Here's how the part is built. I have some questions about the finished solid (model axes, mm). A direction names the side the tool comes from. Round coordinates to 2 decimals unless told otherwise and drop trailing zeros. Loops run counter-clockwise (first coordinate to the right, second up) from the corner with the lowest first, then second, coordinate; pieces in that order, holes last. Notation, with made-up numbers: M -6.75,-12.5 L 28.25,-12.5 A34 cw 28.25,24.5 Z; hole C -33.75,59 d3. An arc over 180 degrees is marked long. Write item = value, one per line. Start each with the question number.
from build123d import *

# Parameters (mm, degrees)
F3_W         = 3.5
F3_H         = 12
F4_DEPTH     = 4
F5_T         = 2
F5_T3_DEPTH  = 6.9649879228
F5_T5_DEPTH  = 12.25
F5_T7_DEPTH  = 10.25
F5_T9_DEPTH  = 5.375
F5_T11_DEPTH = 16
F5_T13_DEPTH = 4.7560633483
F5_T15_DEPTH = 7.5
F5_T17_DEPTH = 5.375
F7_DEPTH     = 25


# Not quite as in the source:
# - a shell that OpenCascade refuses in one call is made with other operations: the cavity is built on its own and cut out


with BuildPart() as f1:
    # F0 (on Front) → F1 (revolve)
    with BuildSketch(Plane.XZ):
        Polygon((60, 2), (0, 14), (0, 0), (60, 0), align=None)
    revolve(axis=Axis((0, 0, 7), (0, 0, -1)))

    # F3 (on offset) → F4 (cut)
    with BuildSketch(Plane.XY.offset(14)):
        Polygon((3.125, -4.125), (3.125, 4.125), (1.75, 4.125), (-1.75, 4.125), (-3.125, 4.125), (-3.125, -4.125), align=None)
        with Locations((0, 10.125)):
            Rectangle(F3_W, F3_H)
    extrude(amount=-F4_DEPTH, mode=Mode.SUBTRACT)

    # F5: shell of thickness 2, made by hand


with BuildPart() as f5_core1:
    # F5_t2: copy of F1
    add(f1.part)

    # the walls: a layer under each face that stays
    f5_faces = [f5_core1.faces().sort_by_distance(p)[0] for p in [
        (-31.5412459886, 0, 7.6917508023),
        (3.125, 0, 11.6875),
        (0, -4.125, 11.5875),
        (-3.125, 0, 11.6875),
        (-2.4375, 4.125, 11.5519137918),
        (-1.75, 10.125, 11.5519137918),
        (0, 16.125, 10.3875),
        (1.75, 10.125, 11.5519137918),
        (2.4375, 4.125, 11.5519137918),
        (-60, 0, 1),
        (0, 6, 10),
    ]]
    thicken(f5_faces, amount=-F5_T, mode=Mode.SUBTRACT)

    # F5_s4 → F5_t3 (cut)
    with BuildSketch(Plane.XY.offset(8)):
        Polygon((3.105, 4.105), (5.125, 4.125), (5.125, 6.125), (3.125, 6.125), align=None)
        Polygon((3.105, -4.105), (5.125, -4.125), (5.125, -6.125), (3.125, -6.125), align=None)
        Polygon((-3.105, -4.105), (-3.125, -6.125), (-5.125, -6.125), (-5.125, -4.125), align=None)
        Polygon((-3.105, 4.105), (-5.125, 4.125), (-5.125, 6.125), (-3.125, 6.125), align=None)
    extrude(amount=F5_T3_DEPTH, mode=Mode.SUBTRACT)

    # F5_s6 → F5_t5 (cut)
    with BuildSketch(Plane.XZ.offset(-6.125)):
        Polygon((3.105, 10.02), (5.125, 10), (5.125, 8), (3.125, 8), align=None)
        Polygon((-3.105, 10.02), (-5.125, 10), (-5.125, 8), (-3.125, 8), align=None)
    extrude(amount=F5_T5_DEPTH, mode=Mode.SUBTRACT)

    # F5_s8 → F5_t7 (cut)
    with BuildSketch(Plane.YZ.offset(-5.125)):
        Polygon((-4.105, 10.02), (-6.125, 10), (-6.125, 8), (-4.125, 8), align=None)
    extrude(amount=F5_T7_DEPTH, mode=Mode.SUBTRACT)

    # F5_s10 → F5_t9 (cut)
    with BuildSketch(Plane.YZ.offset(-5.125)):
        Polygon((4.105, 10.02), (6.125, 10), (6.125, 8), (4.125, 8), align=None)
    extrude(amount=F5_T9_DEPTH, mode=Mode.SUBTRACT)

    # F5_s12 → F5_t11 (cut)
    with BuildSketch(Plane.XZ.offset(-18.125)):
        Polygon((-1.73, 10.02), (-3.75, 10), (-3.75, 8), (-1.75, 8), align=None)
        Polygon((1.73, 10.02), (3.75, 10), (3.75, 8), (1.75, 8), align=None)
    extrude(amount=F5_T11_DEPTH, mode=Mode.SUBTRACT)

    # F5_s14 → F5_t13 (cut)
    with BuildSketch(Plane.XY.offset(8)):
        Polygon((-1.73, 16.105), (-3.75, 16.125), (-3.75, 18.125), (-1.75, 18.125), align=None)
        Polygon((1.73, 16.105), (1.75, 18.125), (3.75, 18.125), (3.75, 16.125), align=None)
    extrude(amount=F5_T13_DEPTH, mode=Mode.SUBTRACT)

    # F5_s16 → F5_t15 (cut)
    with BuildSketch(Plane.YZ.offset(-3.75)):
        Polygon((16.105, 10.02), (18.125, 10), (18.125, 8), (16.125, 8), align=None)
    extrude(amount=F5_T15_DEPTH, mode=Mode.SUBTRACT)

    # F5_s18 → F5_t17 (cut)
    with BuildSketch(Plane.YZ.offset(-0.25)):
        Polygon((4.105, 10.02), (6.125, 10), (6.125, 8), (4.125, 8), align=None)
    extrude(amount=F5_T17_DEPTH, mode=Mode.SUBTRACT)


with BuildPart() as f1_1:
    add(f1.part)

    # what is left inside the walls is the cavity
    f5_cavity = [f5_core1.part.solids().sort_by_distance(p)[0] for p in [
        (0, 19.333333, 0.02),
    ]]
    add(f5_cavity, mode=Mode.SUBTRACT)

    # F6 (on offset) → F7 (cut)
    with BuildSketch(Plane.XY.offset(14)):
        with BuildLine():
            ThreePointArc((5.4351999472, -20.2844423521), (0, -21), (-5.4351999472, -20.2844423521))
            Line((-5.4351999472, -20.2844423521), (-13.9762284355, -52.1599946196))
            ThreePointArc((-13.9762284355, -52.1599946196), (0, -54), (13.9762284355, -52.1599946196))
            Line((13.9762284355, -52.1599946196), (5.4351999472, -20.2844423521))
        make_face()
        with BuildLine():
            ThreePointArc((18.1865334795, -10.5), (14.8492424049, -14.8492424049), (10.5, -18.1865334795))
            Line((10.5, -18.1865334795), (27, -46.7653718044))
            ThreePointArc((27, -46.7653718044), (38.1837661841, -38.1837661841), (46.7653718044, -27))
            Line((46.7653718044, -27), (18.1865334795, -10.5))
        make_face()
        with BuildLine():
            ThreePointArc((20.2844423521, 5.4351999472), (21, 0), (20.2844423521, -5.4351999472))
            Line((20.2844423521, -5.4351999472), (52.1599946196, -13.9762284355))
            ThreePointArc((52.1599946196, -13.9762284355), (54, 0), (52.1599946196, 13.9762284355))
            Line((52.1599946196, 13.9762284355), (20.2844423521, 5.4351999472))
        make_face()
        with BuildLine():
            ThreePointArc((10.5, 18.1865334795), (14.8492424049, 14.8492424049), (18.1865334795, 10.5))
            Line((18.1865334795, 10.5), (46.7653718044, 27))
            ThreePointArc((46.7653718044, 27), (38.1837661841, 38.1837661841), (27, 46.7653718044))
            Line((27, 46.7653718044), (10.5, 18.1865334795))
        make_face()
        with BuildLine():
            ThreePointArc((-5.4351999472, 20.2844423521), (0, 21), (5.4351999472, 20.2844423521))
            Line((5.4351999472, 20.2844423521), (13.9762284355, 52.1599946196))
            ThreePointArc((13.9762284355, 52.1599946196), (0, 54), (-13.9762284355, 52.1599946196))
            Line((-13.9762284355, 52.1599946196), (-5.4351999472, 20.2844423521))
        make_face()
        with BuildLine():
            ThreePointArc((-18.1865334795, 10.5), (-14.8492424049, 14.8492424049), (-10.5, 18.1865334795))
            Line((-10.5, 18.1865334795), (-27, 46.7653718044))
            ThreePointArc((-27, 46.7653718044), (-38.1837661841, 38.1837661841), (-46.7653718044, 27))
            Line((-46.7653718044, 27), (-18.1865334795, 10.5))
        make_face()
        with BuildLine():
            ThreePointArc((-20.2844423521, -5.4351999472), (-21, 0), (-20.2844423521, 5.4351999472))
            Line((-20.2844423521, 5.4351999472), (-52.1599946196, 13.9762284355))
            ThreePointArc((-52.1599946196, 13.9762284355), (-54, 0), (-52.1599946196, -13.9762284355))
            Line((-52.1599946196, -13.9762284355), (-20.2844423521, -5.4351999472))
        make_face()
        with BuildLine():
            ThreePointArc((-10.5, -18.1865334795), (-14.8492424049, -14.8492424049), (-18.1865334795, -10.5))
            Line((-18.1865334795, -10.5), (-46.7653718044, -27))
            ThreePointArc((-46.7653718044, -27), (-38.1837661841, -38.1837661841), (-27, -46.7653718044))
            Line((-27, -46.7653718044), (-10.5, -18.1865334795))
        make_face()
    extrude(amount=-F7_DEPTH, mode=Mode.SUBTRACT)


solid = f1_1.part
Item 1: I want a section at C-C, the plane y = 25. State how many separate pieces and enclosed holes the cut face has, then the cut area to 3 significant figures.
Item 2: I want a section at B-B, the plane x = 0. List the corners of the cut face in (y, z) for me (3 decimals).
Item 3: Will these pins go through, and if not, where does the flat tip stop? pin 1 Ø3 at (x, y) = (36.5, -44.5) entering from +Z; pin 2 Ø6 at (y, z) = (42.5, 10) entering from -X; pin 3 Ø0.9 at (y, z) = (1.5, 9) entering from -X; pin 4 Ø1.5 at (x, z) = (-4, 9.5) entering from +Y.
Item 4: We'd pull the mould along Y, two halves only. Please class faces 3 (the flat face through (-9.726, 36.297, 5.5)), 4 (the flat face through (1.75, 9, 11)), 5 (the cylindrical face through (-59.94, -2.64, 1.01)): released by +Y, released by -Y, zero draft, split by the parting line, or undercut.
Item 5: I want a section at A-A, the plane y = 0. List the corners of the cut face in (x, z) for me (3 decimals), then the cut area to 3 significant figures.
Item 6: For faces 1 (the flat face through (-1.75, 9, 11)), 2 (the flat face through (-32.543, 18.788, 5.5)), which set-ups out of +Z, -Z, +X, -X, +Y, -Y let a thin tool reach every point of the face, with its end or its side?
Item 7: Please list where these lines run through material, in increasing order: line 1 (Y direction, x = 0, z = 0.25); line 2 (Z direction, x = -45.5, y = -39). Write a range as [from, to].
Worked out:
q1.separate_pieces = 4
q1.enclosed_holes = 0
q1.area = 78.1 mm2
q2.outline = M -60,0 L -58,0 L -58,0.36 L -54,1.16 L -54,3.2 L -60,2 Z; M -21,7.76 L -6.125,10.735 L -6.125,8 L 18.125,8 L 18.125,8.335 L 21,7.76 L 21,9.8 L 16.125,10.775 L 16.125,10 L -4.125,10 L -4.125,13.175 L -21,9.8 Z; M 54,1.16 L 58,0.36 L 58,0 L 60,0 L 60,2 L 54,3.2 Z
q3.pin_1 = 2.79
q3.pin_2 = through
q3.pin_3 = -20.97
q3.pin_4 = 20.75
q4.face_3 = undercut
q4.face_4 = undercut
q4.face_5 = split by the parting line
q5.outline = M -60,0 L -58,0 L -58,0.36 L -54,1.16 L -54,3.2 L -60,2 Z; M -21,7.76 L -5.125,10.935 L -5.125,8 L 5.125,8 L 5.125,10.935 L 21,7.76 L 21,9.8 L 3.125,13.375 L 3.125,10 L -3.125,10 L -3.125,13.375 L -21,9.8 Z; M 54,1.16 L 58,0.36 L 58,0 L 60,0 L 60,2 L 54,3.2 Z
q5.area = 123 mm2
q6.face_1 = +Z
q6.face_2 = +Z, -Z
q7.line_1 = [-60, -58], [58, 60]
q7.line_2 = [0, 2.01]
